```python
from build123d import *

# Parameters (mm, degrees)
F0_R     = 3.5052
F1_DEPTH = 6.35
F3_DEPTH = 2.54


with BuildPart() as f1:
    # F0 (on Front) → F1 (new body)
    with BuildSketch(Plane.XZ):
        Polygon((-11.3974893229, 44.2205731771), (-49.2346257812, -48.5394), (-36.2149429687, -48.5394), (-25.533746875, -21.4045270833), (16.7275536458, -21.4045270833), (27.3244799479, -48.5394), (40.1545557292, -48.5394), (2.9073078125, 44.2205731771), align=None)
        with Locations((-39.6848618984, -41.1395020783)):
            Circle(F0_R, mode=Mode.SUBTRACT)
        with Locations((30.8506265283, -41.1395020783)):
            Circle(F0_R, mode=Mode.SUBTRACT)
        with Locations((-4.3683550321, -16.2198841572)):
            Circle(F0_R, mode=Mode.SUBTRACT)
        with BuildLine():
            Line((-4.9929851562, 32.9073536458), (-4.4030966146, 34.7402216146))
            Line((-4.4030966146, 34.7402216146), (-2.6334309896, 29.2837526042))
            add(Edge.make_bspline(
                [(1.0533723958, 19.0028380208), (-0.7794955729, 23.5534067708), (-2.6334309896, 29.2837526042)],
                knots=[0, 0, 0, 1, 1, 1], degree=2))
            Line((1.0533723958, 19.0028380208), (12.9775479167, -11.6081638021))
            Line((12.9775479167, -11.6081638021), (-21.7205388021, -11.6081638021))
            Line((-21.7205388021, -11.6081638021), (-9.8806330729, 18.8764333333))
            add(Edge.make_bspline(
                [(-4.9929851562, 32.9073536458), (-6.6573135417, 27.4298171875), (-9.8806330729, 18.8764333333)],
                knots=[0, 0, 0, 1, 1, 1], degree=2))
        make_face(mode=Mode.SUBTRACT)
        with BuildLine():
            Line((-49.2346257812, -48.5394), (-49.5085026042, -48.5394))
            Line((-49.5085026042, -48.5394), (-49.5085026042, -64.4144))
            ThreePointArc((-49.5085026042, -64.4144), (-39.9835026042, -73.9394), (-49.5085026042, -83.4644))
            Line((-49.5085026042, -83.4644), (-49.5085026042, -99.3394))
            Line((-49.5085026042, -99.3394), (52.0914973958, -99.3394))
            Line((52.0914973958, -99.3394), (52.0914973958, -83.3374))
            ThreePointArc((52.0914973958, -83.3374), (61.4894973958, -73.9394), (52.0914973958, -64.5414))
            Line((52.0914973958, -64.5414), (52.0914973958, -48.5394))
            Line((52.0914973958, -48.5394), (40.1545557292, -48.5394))
            Line((40.1545557292, -48.5394), (27.3244799479, -48.5394))
            Line((27.3244799479, -48.5394), (-36.2149429687, -48.5394))
            Line((-36.2149429687, -48.5394), (-49.2346257812, -48.5394))
        make_face()
    extrude(amount=F1_DEPTH)

    # F2 (on face) → F3 (cut)
    with BuildSketch(Plane.XZ.offset(6.35)):
        with BuildLine():
            ThreePointArc((-6.7838939248, -18.7598839402), (-7.8735550321, -16.2198841572), (-6.7838939248, -13.6798843741))
            Line((-6.7838939248, -13.6798843741), (-31.0344029758, -13.6798843741))
            Line((-31.0344029758, -13.6798843741), (-41.1044888823, -37.9346485299))
            ThreePointArc((-41.1044888823, -37.9346485299), (-38.340810813, -37.902226415), (-36.4127835596, -39.882549261))
            Line((-36.4127835596, -39.882549261), (-27.6430815337, -18.7598839402))
            Line((-27.6430815337, -18.7598839402), (-6.7838939248, -18.7598839402))
        make_face()
        with BuildLine():
            ThreePointArc((27.5828955219, -39.8712903019), (29.5177289249, -37.8976182095), (32.2812779405, -37.9395546449))
            Line((32.2812779405, -37.9395546449), (22.3069365793, -13.6798843741))
            Line((22.3069365793, -13.6798843741), (-1.9528161394, -13.6798843741))
            ThreePointArc((-1.9528161394, -13.6798843741), (-1.1470684904, -14.8379507085), (-0.8631550321, -16.2198841572))
            ThreePointArc((-0.8631550321, -16.2198841572), (-1.1470684904, -17.6018176059), (-1.9528161394, -18.7598839402))
            Line((-1.9528161394, -18.7598839402), (18.9029600028, -18.7598839402))
            Line((18.9029600028, -18.7598839402), (27.5828955219, -39.8712903019))
        make_face()
        with BuildLine():
            Line((33.3906265283, -70.1294), (33.3906265283, -43.5550407429))
            ThreePointArc((33.3906265283, -43.5550407429), (30.8506265283, -44.6447020783), (28.3106265283, -43.5550407429))
            Line((28.3106265283, -43.5550407429), (28.3106265283, -70.1294))
            Line((28.3106265283, -70.1294), (-40.7786959053, -70.1294))
            ThreePointArc((-40.7786959053, -70.1294), (-39.9835026042, -73.9394), (-40.7786959053, -77.7494))
            Line((-40.7786959053, -77.7494), (60.6825569347, -77.7494))
            ThreePointArc((60.6825569347, -77.7494), (61.4894973958, -73.9394), (60.6825569347, -70.1294))
            Line((60.6825569347, -70.1294), (33.3906265283, -70.1294))
        make_face()
    extrude(amount=-F3_DEPTH, mode=Mode.SUBTRACT)


solid = f1.part
```
Design review of the part built by this model. Coordinates are the model's own, in mm. A direction names the side the tool comes from. Coordinates: 2 decimals unless noted, no trailing zeros. Order: outer loops, then holes, each group sorted by start corner. A loop starts at its lowest first (then second) coordinate and runs counter-clockwise, first axis right, second up. Notation, with made-up numbers: (74.5, 68.5) - (90.5, 68.5) arc R25 cw to (90.5, 99.5) - close; hole circle Ø3 at (41.25, -34.75). An arc over 180 degrees is marked (long way). One line per question, with ' | ' between items.
Q1. Consider section D-D, the plane x = -20. Give the boundary of the cut face in (y, z).
Answer key:
outline: (-6.35, -99.34) - (0, -99.34) - (0, -48.54) - (-6.35, -48.54) - (-6.35, -70.13) - (-3.81, -70.13) - (-3.81, -77.75) - (-6.35, -77.75) - close; (-6.35, -21.4) - (0, -21.4) - (0, -11.61) - (-6.35, -11.61) - (-6.35, -13.68) - (-3.81, -13.68) - (-3.81, -18.76) - (-6.35, -18.76) - close; (-6.35, -7.18) - (0, -7.18) - (0, 23.13) - (-6.35, 23.13) - close
Q2. Consider section B-B, the plane z = -34. Give the boundary of the cut face in (x, y), then the cut area to 3 significant figures.
Answer key:
outline: (-43.3, -6.35) - (-39.47, -6.35) - (-39.47, -3.81) - (-33.97, -3.81) - (-33.97, -6.35) - (-30.49, -6.35) - (-30.49, 0) - (-43.3, 0) - close; (21.65, -6.35) - (25.17, -6.35) - (25.17, -3.81) - (30.66, -3.81) - (30.66, -6.35) - (34.32, -6.35) - (34.32, 0) - (21.65, 0) - close | area: 134 mm2
Q3. Clearance check with flat-ended pins moving along their axes: pin 1 Ø0.8 at (y, z) = (-4.5, -52.5) entering from +X; pin 2 Ø4 at (x, z) = (35, -26.5) entering from +Y; pin 3 Ø0.8 at (x, y) = (-20.5, -5.5) entering from +Z; pin 4 Ø3 at (y, z) = (-2.5, 8.5) entering from -X. State where each tip first meets the part, or that it passes through.
Answer key:
pin 1: stops at x = 52.09 | pin 2: passes through | pin 3: stops at z = 22.89 | pin 4: stops at x = -26.58
Q4. To check wall thickness, follow line 1 along Z through (x, y) = (45, -5.5); line 2 along Z through (x, y) = (-24, -5.25); line 3 along X through (y, z) = (-1.75, -41). State the ranges of each line that lie inside material, in increasing order.
Answer key:
line 1: z = -99.34 to -77.75, -70.13 to -48.54 | line 2: z = -99.34 to -77.75, -70.13 to -48.54, -21.4 to -18.76, -13.68 to 13.32 | line 3: x = -46.16 to -43.19, -36.18 to -33.25, 24.38 to 27.35, 34.35 to 37.13
Q5. The part is to be moulded in two halves that separate along Z. For faces 4 (the cylindrical face through (61.487, -3.131, -74.146)), 5 (the flat face through (52.091, -3, -57)), 6 (the cylindrical face through (-1.025, -2.425, -15.167)), 7 (the flat face through (21.792, -3.131, -2.809)), say which applies: +Z half, -Z half, draft (parallel to the pull), parting line (faces both ways), or undercut.
Answer key:
face 4: parting line | face 5: draft | face 6: undercut | face 7: +Z half
Q6. Consider section A-A, the plane x = 4.5. Give the boundary of the cut face in (y, z), then the cut area to 3 significant figures.
Answer key:
outline: (-6.35, -99.34) - (0, -99.34) - (0, -48.54) - (-6.35, -48.54) - (-6.35, -70.13) - (-3.81, -70.13) - (-3.81, -77.75) - (-6.35, -77.75) - close; (-6.35, -21.4) - (0, -21.4) - (0, -11.61) - (-6.35, -11.61) - (-6.35, -13.68) - (-3.81, -13.68) - (-3.81, -18.76) - (-6.35, -18.76) - close; (-6.35, 10.15) - (0, 10.15) - (0, 40.25) - (-6.35, 40.25) - close | area: 544 mm2
Q7. Consider section C-C, the plane y = -2.75. Give the number of separate pieces and of enclosed holes in the cut face, then the cut area to 3 significant figures.
Answer key:
separate pieces: 1 | enclosed holes: 5 | area: 7,640 mm2
Q8. For faces 1 (the flat face through (1, -3, -99.339)), 2 (the flat face through (-4, -3, -48.539)), 3 (the flat face through (-32.1, -5.1, -29.5)), list the 3-axis set-ups (+Z, -Z, +X, -X, +Y, -Y) from which the entire face can be reached by the end or side of a thin tool; tool diameter is ignored.
Answer key:
face 1: -Z, +X, -X, +Y, -Y | face 2: +Y, -Y | face 3: -Y
